```python
from build123d import *

# Parameters (mm, degrees)
SKETCH_W        = 100
SKETCH_H        = 50
SKETCH_R        = 2.6
PAD_DEPTH       = 5
SKETCH001_W     = 50
SKETCH001_H     = 30
PAD001_DEPTH    = 30
SKETCH003_R     = 5.75
POCKET001_DEPTH = 12
SKETCH004_R     = 3
POCKET_DEPTH    = 34
SKETCH005_R     = 3
POCKET002_DEPTH = 5
SKETCH006_R     = 4.31
POCKET003_DEPTH = 13
FILLET_R        = 10


with BuildPart() as part:
    # Sketch → Pad (new body)
    with BuildSketch(Plane.YZ):
        Rectangle(SKETCH_W, SKETCH_H)
        with Locations((-30, 15)):
            Circle(SKETCH_R, mode=Mode.SUBTRACT)
        with Locations((-30, -15)):
            Circle(SKETCH_R, mode=Mode.SUBTRACT)
    extrude(amount=PAD_DEPTH)

    # Sketch001 (on Face8 of Pad) → Pad001 (join)
    with BuildSketch(Plane.YZ.offset(5)):
        with Locations((25, 0)):
            Rectangle(SKETCH001_W, SKETCH001_H)
    extrude(amount=PAD001_DEPTH)

    # Sketch003 → Pocket001 (cut)
    with BuildSketch(Plane(origin=(0, 0, 0), x_dir=(0, 1, 0), z_dir=(-1, 0, 0))):
        with Locations((25, 0)):
            Circle(SKETCH003_R)
    extrude(amount=-POCKET001_DEPTH, mode=Mode.SUBTRACT)

    # Sketch004 (on DatumPlane) → Pocket (cut)
    with BuildSketch(Plane(origin=(0, 8, 0), x_dir=(0, 0, -1), z_dir=(0, -1, 0))):
        with Locations((0, 20)):
            Circle(SKETCH004_R)
    extrude(amount=-POCKET_DEPTH, mode=Mode.SUBTRACT)

    # Sketch005 (on Face15 of Pocket) → Pocket002 (cut)
    with BuildSketch(Plane(origin=(12, 0, 0), x_dir=(0, 1, 0), z_dir=(-1, 0, 0))):
        with Locations((25, 0)):
            Circle(SKETCH005_R)
    extrude(amount=-POCKET002_DEPTH, mode=Mode.SUBTRACT)

    # Sketch006 (on Face14 of Pocket002) → Pocket003 (cut)
    with BuildSketch(Plane.YZ.offset(35)):
        with Locations((10, 0)):
            Circle(SKETCH006_R)
        with Locations((40, 0)):
            Circle(SKETCH006_R)
    extrude(amount=-POCKET003_DEPTH, mode=Mode.SUBTRACT)

    # Fillet
    fillet_edges = [part.edges().sort_by_distance(p)[0] for p in [
        (2.5, -50, 25),
        (2.5, 50, -25),
        (2.5, 50, 25),
        (2.5, -50, -25),
    ]]
    fillet(fillet_edges, radius=FILLET_R)


solid = part.part
```
Work out the finished part from the listing and answer in its coordinate system (mm). A direction names the side the tool comes from. Round coordinates to 2 decimals unless told otherwise and drop trailing zeros. Loops run counter-clockwise (first coordinate to the right, second up) from the corner with the lowest first, then second, coordinate; pieces in that order, holes last.
(1) The part is cut by section D-D, the plane z = -8. Give the vertices of the cut face in (x, y), and give its area (3 significant figures).
Computed values:
outline: (0, -50) - (5, -50) - (5, 0) - (35, 0) - (35, 50) - (0, 50) - close
area: 2,000 mm2
(2) For faces 1 (the flat face through (0, -1, 0)), 2 (the flat face through (20, 42, 0)), 3 (the cylindrical face through (28.591, 44.111, 1.295)), 4 (the flat face through (5, -12, 0)), 5 (the flat face through (12, 27.5, 2.5)), determine the directions among +Z, -Z, +X, -X, +Y, -Y from which every point of the face is accessible in a straight line to the end or side of a thin tool.
Computed values:
face 1: +Z, -Z, -X, +Y, -Y
face 2: none
face 3: +X
face 4: +X, -Y
face 5: -X
(3) The mould has two halves that part along Y. Classify faces 6 (the flat face through (20, 25, 15)), 7 (the cylindrical face through (2.54, 46.99, 22.15)), 8 (the flat face through (22, 43, 0)), 9 (the flat face through (22, 7.85, 0.06)): pulls with the +Y half, pulls with the -Y half, needs draft (parallel to the pull), parting line crosses it, or undercut.
Computed values:
face 6: needs draft
face 7: pulls with the +Y half
face 8: undercut
face 9: undercut
(4) Find the intervals of material crossed by L1, parallel to Z at x = 20, y = 29; L2, parallel to Y at x = 8, z = 0; L3, parallel to X at y = -40, z = -15, in increasing order.
Computed values:
L1: z = -15 to -3, 3 to 15
L2: y = 0 to 19.25, 30.75 to 50
L3: x = 0 to 5
(5) The part is cut by section C-C, the plane x = 25. Give the vertices of the cut face in (y, z), and give its area (3 significant figures).
Computed values:
outline: (0, -15) - (50, -15) - (50, 15) - (0, 15) - close; hole circle Ø8.62 at (10, 0); hole circle Ø8.62 at (40, 0)
area: 1,380 mm2
(6) The part is cut by section A-A, the plane y = -30. Give the vertices of the cut face in (x, z), and give its area (3 significant figures).
Computed values:
outline: (0, -25) - (5, -25) - (5, -17.6) - (0, -17.6) - close; (0, -12.4) - (5, -12.4) - (5, 12.4) - (0, 12.4) - close; (0, 17.6) - (5, 17.6) - (5, 25) - (0, 25) - close
area: 198 mm2
(7) The part is cut by section B-B, the plane x = 7.5. Give the vertices of the cut face in (y, z), and give its area (3 significant figures).
Computed values:
outline: (0, -15) - (50, -15) - (50, 15) - (0, 15) - close; hole circle Ø11.5 at (25, 0)
area: 1,400 mm2
(8) Each of these flat-tipped pins is pushed along its axis until it touches: P1, Ø8, axis at x = 29.5, y = 16, coming from the +Z side; P2, Ø4, axis at y = 42, z = -1.5, coming from the +X side; P3, Ø4.5, axis at y = -30, z = -15, coming from the +X side; P4, Ø2.5, axis at y = 26, z = 2, coming from the -X side. Where does it stop, or does it pass through?
Computed values:
P1: stops at z = 15
P2: stops at x = 35
P3: passes through
P4: stops at x = 12
